For this review, use the dimensioned drawing (mm, ordinates from the lowest corner) and the shaded views. A direction names the side the tool comes from. Coordinates: 2 decimals unless noted, no trailing zeros. Write each loop counter-clockwise with the first axis right and the second up, starting at its lowest first coordinate (ties: lowest second). Pieces come first, ordered by that corner, then holes. Notation, with made-up numbers: (-5, -23.5) - (18, -23.5) arc R19 ccw to (18, -8.5) - close; hole circle Ø4 at (26.25, 68). An arc over 180 degrees is marked (long way). One line per item, written item: value.
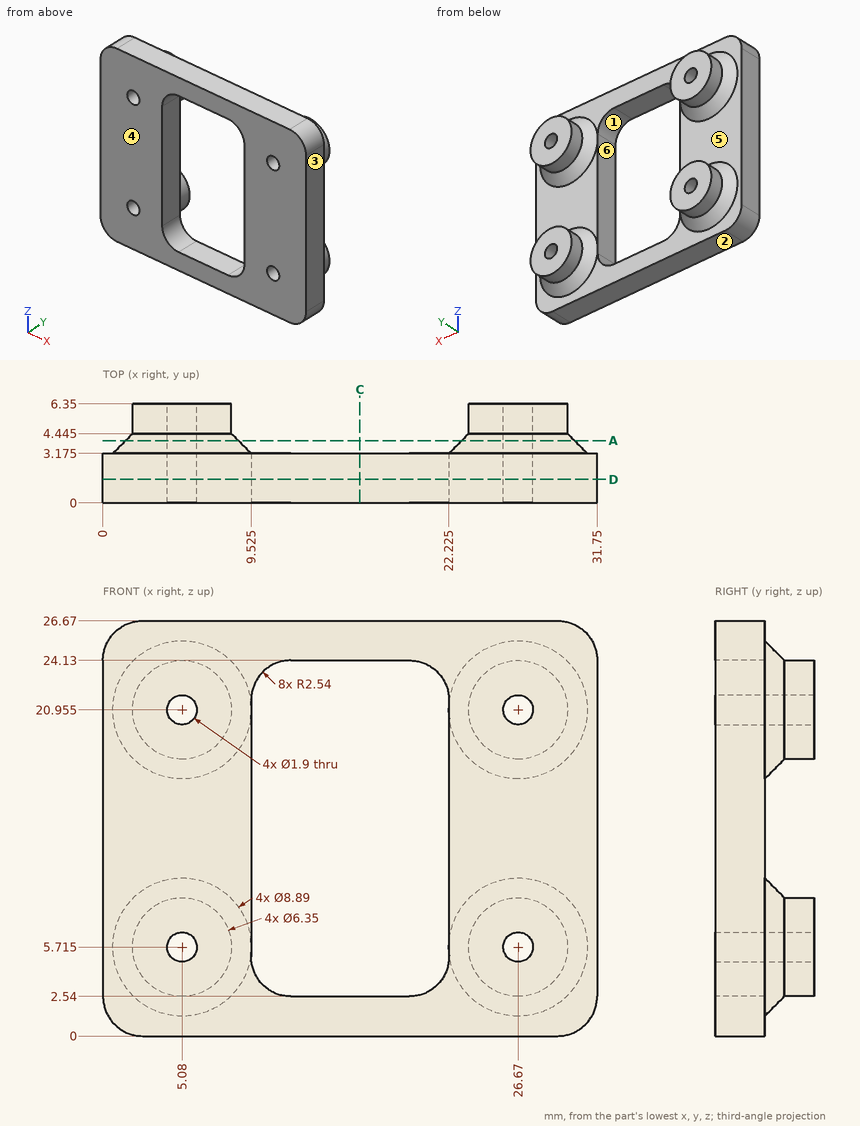
1. For the marked faces 4, 5 and 6, list the 3-axis set-ups (+Z, -Z, +X, -X, +Y, -Y) from which the entire face can be reached by the end or side of a thin tool; tool diameter is ignored.
Answer block:
face 4: +Z, -Z, +X, -X, -Y
face 5: +Y
face 6: +Y, -Y
2. Consider section A-A, the plane y = 4. Give the number of separate pieces and of enclosed holes in the cut face, then the cut area to 3 significant figures.
Answer block:
separate pieces: 4
enclosed holes: 4
area: 153 mm^2
3. Wall thickness on line 1 along Z through (x, y) = (26.67, 5) (3 decimals); line 2 along Z through (x, y) = (18, 3); line 3 along X through (y, z) = (1, 17.5) (3 decimals): over which ranges is each line inside the solid? List them lowest first.
Answer block:
line 1: z = 2.54 to 4.765, 6.665 to 8.89, 17.78 to 20.005, 21.905 to 24.13
line 2: z = 0 to 2.54, 24.13 to 26.67
line 3: x = 0 to 9.525, 22.225 to 31.75
4. Consider section D-D, the plane y = 1.5. Write out the cut boundary in (x, z) (3 decimals).
Answer block:
outline: (0, 2.54) arc R2.54 ccw to (2.54, 0) - (29.21, 0) arc R2.54 ccw to (31.75, 2.54) - (31.75, 24.13) arc R2.54 ccw to (29.21, 26.67) - (2.54, 26.67) arc R2.54 ccw to (0, 24.13) - close; hole circle Ø1.9 at (5.08, 5.715); hole circle Ø1.9 at (5.08, 20.955); hole (9.525, 5.08) arc R2.54 ccw to (12.065, 2.54) - (19.685, 2.54) arc R2.54 ccw to (22.225, 5.08) - (22.225, 21.59) arc R2.54 ccw to (19.685, 24.13) - (12.065, 24.13) arc R2.54 ccw to (9.525, 21.59) - close; hole circle Ø1.9 at (26.67, 5.715); hole circle Ø1.9 at (26.67, 20.955)
5. Consider section C-C, the plane x = 16.5. Write out the cut boundary in (y, z) (3 decimals).
Answer block:
outline: (0, 0) - (3.175, 0) - (3.175, 2.54) - (0, 2.54) - close; (0, 24.13) - (3.175, 24.13) - (3.175, 26.67) - (0, 26.67) - close
6. Insertion check: pin 1 Ø8 at (x, z) = (20, 9) entering from +Y (1 decimal); pin 2 Ø1.5 at (y, z) = (5, 4) entering from -X (1 decimal). Each pin has a flat end and moves straight along its axis. Give the tip position at first contact, or say it passes through.
Answer block:
pin 1: stops at y = 4.2
pin 2: stops at x = 2.1
7. Mouldability with a two-part tool opening along Z and no side actions: class the marked faces 1, 2 and 3 as released by +Z, released by -Z, zero draft, split by the parting line, or undercut.
Answer block:
face 1: undercut
face 2: released by -Z
face 3: zero draft
